The listing builds one solid part. Answer for the finished solid, in the listing's coordinates (mm). A direction names the side the tool comes from. Give positions to 0.01 mm unless a question says otherwise; leave off trailing zeros. Write each loop counter-clockwise with the first axis right and the second up, starting at its lowest first coordinate (ties: lowest second). Pieces come first, ordered by that corner, then holes. Notation, with made-up numbers: (66, -16) -> (85, -16) arc R19 cw to (85, -9) -> close; hole circle Ø1 at (71.25, -21.75). An arc over 180 degrees is marked (long way). Put each result on its own line as item: value. Start each with the question number.
1) For faces 4 (the flat face through (8.699, 13, 8)), 5 (the flat face through (-13, 9.5, -12)), 6 (the flat face through (-13, 5, 6.329)), determine the directions among +Z, -Z, +X, -X, +Y, -Y from which every point of the face is accessible in a straight line to the end or side of a thin tool.
2) A cutting plane is placed at A-A (z = -10.5). Write down the section's boundary in (x, y), then the cut area to 3 significant figures.
3) A cutting plane is placed at C-C (z = 5.5). Write down the section's boundary in (x, y), then the cut area to 3 significant figures.
4) Find the intervals of material crossed by line 1 along Z through (x, y) = (-1.5, 9); line 2 along Z through (x, y) = (-6, 18.5); line 3 along X through (y, z) = (4.5, -12.5), in increasing order. Write a range as from..to.
5) A cutting plane is placed at B-B (x = -23.5). Write down the section's boundary in (y, z), then the cut area to 3 significant figures.
6) For a pull along Y with two mould halves and no side action, classify faces 1 (the flat face through (12, 2, -7)), 2 (the cylindrical face through (6.674, 30.573, -1.74)), 3 (the flat face through (4.699, 4, -14)) as released by +Y, released by -Y, zero draft, split by the parting line, or undercut.
7) Flat-ended cylindrical pins translate along their axes: pin 1 Ø10 at (x, z) = (18, 10.5) entering from +Y; pin 2 Ø1.5 at (x, z) = (-13, 2.5) entering from -Y; pin 3 Ø8 at (x, y) = (11.5, 25.5) entering from +Z. Find the tip coordinate at first contact, or state that the pin passes through.
from build123d import *

# Parameters (mm, degrees)
SKETCH1_W           = 48
SKETCH1_H           = 27.75
BOSS_EXTRUDE1_DEPTH = 31
CUT_EXTRUDE1_DEPTH  = 36
SKETCH3_W           = 22
SKETCH3_H           = 25.75
CUT_EXTRUDE2_DEPTH  = 29
CUT_EXTRUDE3_DEPTH  = 45.957983893
BOSS_EXTRUDE2_START = -26
SKETCH5_W           = 27.75
SKETCH5_H           = 17
BOSS_EXTRUDE2_DEPTH = 41
SKETCH10_W          = 27.75
SKETCH10_H          = 23
BOSS_EXTRUDE4_DEPTH = 8
CHAMFER1_SIZE       = 38
CHAMFER1_SIZE2      = 10
FILLET1_R           = 10
SKETCH6_W           = 9
SKETCH6_H           = 9.5
CUT_EXTRUDE4_DEPTH  = 8
BOSS_EXTRUDE3_DEPTH = 18
SKETCH8_R           = 1.375
CUT_EXTRUDE5_DEPTH  = 17
SKETCH9_W           = 6
SKETCH9_H           = 10
CUT_EXTRUDE6_DEPTH  = 9


with BuildPart() as part:
    # Sketch1 → Boss-Extrude1 (new body)
    with BuildSketch(Plane(origin=(0, 0, 0), x_dir=(1, 0, 0), z_dir=(0, 1, 0))):
        with Locations((6.698630137, 1.546232877)):
            Rectangle(SKETCH1_W, SKETCH1_H)
    extrude(amount=BOSS_EXTRUDE1_DEPTH)

    # Sketch2 → Cut-Extrude1 (cut)
    with BuildSketch(Plane.ZY.offset(17.301369863)):
        Polygon((-7.921232877, 25.25), (4.828767123, 25.25), (4.828767123, 2), (2.703767123, 2), (2.703767123, 0), (-5.796232877, 0), (-5.796232877, 2), (-7.921232877, 2), align=None)
    extrude(amount=-CUT_EXTRUDE1_DEPTH, mode=Mode.SUBTRACT)

    # Sketch3 → Cut-Extrude2 (cut)
    with BuildSketch(Plane(origin=(0, 31, 0), x_dir=(1, 0, 0), z_dir=(0, 1, 0))):
        with Locations((19.698630137, 1.546232877)):
            Rectangle(SKETCH3_W, SKETCH3_H)
    extrude(amount=-CUT_EXTRUDE2_DEPTH, mode=Mode.SUBTRACT)

    # Sketch4 → Cut-Extrude3 (cut, through all)
    with BuildSketch(Plane(origin=(0, 2, 0), x_dir=(1, 0, 0), z_dir=(0, 1, 0))):
        with BuildLine():
            Line((20.698630137, -1.953767123), (18.698630137, -1.953767123))
            ThreePointArc((18.698630137, -1.953767123), (15.198630137, 1.546232877), (18.698630137, 5.046232877))
            Line((18.698630137, 5.046232877), (20.698630137, 5.046232877))
            ThreePointArc((20.698630137, 5.046232877), (24.198630137, 1.546232877), (20.698630137, -1.953767123))
        make_face()
    extrude(amount=-CUT_EXTRUDE3_DEPTH, mode=Mode.SUBTRACT)

    # Sketch5 → Boss-Extrude2 (add)
    with BuildSketch(Plane.ZY.offset(17.301369863).offset(BOSS_EXTRUDE2_START)):
        with Locations((-1.546232877, 33.75)):
            Rectangle(SKETCH5_W, SKETCH5_H)
    extrude(amount=BOSS_EXTRUDE2_DEPTH)

    # Sketch10 → Boss-Extrude4 (add)
    with BuildSketch(Plane.ZY.offset(32.301369863)):
        with Locations((-1.546232877, 30.75)):
            Rectangle(SKETCH10_W, SKETCH10_H)
    extrude(amount=-BOSS_EXTRUDE4_DEPTH)

    # Chamfer1
    chamfer1_edges = [part.edges().sort_by_distance(p)[0] for p in [
        (8.698630137, 42.25, -1.546232877),
    ]]
    chamfer1_side = [part.faces().sort_by_distance(p)[0] for p in [
        (-11.801369863, 42.25, -1.546232877),
    ]]
    chamfer(chamfer1_edges, length=CHAMFER1_SIZE, length2=CHAMFER1_SIZE2, reference=chamfer1_side[0])

    # Fillet1
    # the kernel refuses this fillet: 10 mm, written as the material it takes off along each edge
    with BuildSketch(Plane(origin=(30.698630137, 31, -40.421232877), x_dir=(-1, 0, 0), z_dir=(0, 0, 1))) as fillet1_piece_1:
        with BuildLine():
            CenterArc((FILLET1_R, FILLET1_R), FILLET1_R, 180, 90)
            Line((0, FILLET1_R), (0, 0))
            Line((0, 0), (FILLET1_R, 0))
        make_face()
    extrude(amount=51, mode=Mode.SUBTRACT)
    with BuildSketch(Plane(origin=(30.698630137, 31, -13.671232877), x_dir=(0, -1, 0), z_dir=(0, 0, 1))) as fillet1_piece_2:
        with BuildLine():
            CenterArc((FILLET1_R, -FILLET1_R), FILLET1_R, 90, 90)
            Line((0, -FILLET1_R), (0, 0))
            Line((0, 0), (FILLET1_R, 0))
        make_face()
    extrude(amount=51, mode=Mode.SUBTRACT)
    with BuildSketch(Plane(origin=(8.698630137, 32.25, -34.693446961), x_dir=(-0.9670745372626461, 0.25449329927964454, 0), z_dir=(0, 0, 1))) as fillet1_piece_3_section:
        with BuildLine():
            CenterArc((FILLET1_R * 0.770888563389, FILLET1_R), FILLET1_R, 194.743562836, 75.256437164)
            Line((-FILLET1_R * 0.196185973874, FILLET1_R * 0.74550670072), (0, 0))
            Line((0, 0), (FILLET1_R * 0.770888563389, 0))
        make_face()
    fillet1_piece_3 = extrude(amount=66.294428169, mode=Mode.PRIVATE)
    fillet1_piece_3 = split(fillet1_piece_3, bisect_by=Plane(origin=(6.418470389, 31, -14.921232877), z_dir=(0, 1, 0)), keep=Keep.TOP, mode=Mode.PRIVATE)
    add(fillet1_piece_3, mode=Mode.SUBTRACT)
    with BuildSketch(Plane(origin=(8.698630137, 32.25, -34.693446961), x_dir=(-0.9670745372626461, 0.25449329927964454, 0), z_dir=(0, 0, 1))) as fillet1_piece_4_section:
        with BuildLine():
            CenterArc((FILLET1_R * 0.770888563389, FILLET1_R), FILLET1_R, 194.743562836, 75.256437164)
            Line((-FILLET1_R * 0.196185973874, FILLET1_R * 0.74550670072), (0, 0))
            Line((0, 0), (FILLET1_R * 0.770888563389, 0))
        make_face()
    fillet1_piece_4 = extrude(amount=66.294428169, mode=Mode.PRIVATE)
    fillet1_piece_4 = split(fillet1_piece_4, bisect_by=Plane(origin=(8.005221355, 29.431341636, -14.421232877), z_dir=(0, 0, 1)), keep=Keep.TOP, mode=Mode.PRIVATE)
    fillet1_piece_4 = split(fillet1_piece_4, bisect_by=Plane(origin=(8.005221355, 29.431341636, 11.328767123), z_dir=(0, 0, -1)), keep=Keep.TOP, mode=Mode.PRIVATE)
    add(fillet1_piece_4, mode=Mode.SUBTRACT)

    # Sketch6 → Cut-Extrude4 (cut)
    with BuildSketch(Plane.ZY.offset(17.301369863)):
        with Locations((10.828767123, 4.75)):
            Rectangle(SKETCH6_W, SKETCH6_H)
    cut_extrude4 = extrude(amount=-CUT_EXTRUDE4_DEPTH, mode=Mode.SUBTRACT)

    # Sketch7 → Boss-Extrude3 (add)
    with BuildSketch(Plane.ZY.offset(9.301369863)):
        Polygon((12.328767123, 0), (12.328767123, 9.5), (12.328767123, 14.5), (15.328767123, 14.5), (15.328767123, 9.5), (15.328767123, 0), (15.328767123, -0.5), (6.328767123, -0.5), (6.328767123, 0), align=None)
    boss_extrude3 = extrude(amount=-BOSS_EXTRUDE3_DEPTH)

    # Sketch8 → Cut-Extrude5 (cut)
    with BuildSketch(Plane.ZY.offset(9.301369863)):
        with Locations((12.328767123, 2)):
            Circle(SKETCH8_R)
    cut_extrude5 = extrude(amount=-CUT_EXTRUDE5_DEPTH, mode=Mode.SUBTRACT)

    # Sketch9 → Cut-Extrude6 (cut)
    with BuildSketch(Plane.XY.offset(15.328767123)):
        with Locations((1.698630137, 4.5)):
            Rectangle(SKETCH9_W, SKETCH9_H)
    cut_extrude6 = extrude(amount=-CUT_EXTRUDE6_DEPTH, mode=Mode.SUBTRACT)

    # Mirror1: Cut-Extrude4, Boss-Extrude3, Cut-Extrude5, Cut-Extrude6 across plane
    add(cut_extrude4.mirror(Plane.XY.offset(-1.546232877)), mode=Mode.SUBTRACT)
    add(boss_extrude3.mirror(Plane.XY.offset(-1.546232877)))
    add(cut_extrude5.mirror(Plane.XY.offset(-1.546232877)), mode=Mode.SUBTRACT)
    add(cut_extrude6.mirror(Plane.XY.offset(-1.546232877)), mode=Mode.SUBTRACT)


solid = part.part
Reply:
1. face 4: +X, +Y
1. face 5: -Z, -X, -Y
1. face 6: +Z, -X, -Y
2. outline: (-32.3, 19.25) -> (-24.3, 19.25) -> (-24.3, 25.25) -> (-17.3, 25.25) -> (-17.3, 9.5) -> (-9.3, 9.5) -> (-9.3, -0.5) -> (-1.3, -0.5) -> (-1.3, 9.5) -> (4.7, 9.5) -> (4.7, -0.5) -> (8.7, -0.5) -> (8.7, 0) -> (30.7, 0) -> (30.7, 2) -> (8.7, 2) -> (8.7, 24.54) arc R10 ccw to (1.24, 34.21) -> (-29.3, 42.25) -> (-32.3, 42.25) -> close
2. area: 1,120 mm2
3. outline: (-32.3, 19.25) -> (-24.3, 19.25) -> (-24.3, 25.25) -> (-17.3, 25.25) -> (-17.3, 0) -> (30.7, 0) -> (30.7, 2) -> (8.7, 2) -> (8.7, 24.54) arc R10 ccw to (1.24, 34.21) -> (-29.3, 42.25) -> (-32.3, 42.25) -> close
3. area: 1,240 mm2
4. line 1: z = -18.42..-7.92, 4.83..15.33
4. line 2: z = -15.42..-7.92, 4.83..12.33
4. line 3: x = -9.3..-1.3, 4.7..8.7
5. outline: (25.25, -15.42) -> (40.72, -15.42) -> (40.72, 12.33) -> (25.25, 12.33) -> close
5. area: 429 mm2
6. face 1: undercut
6. face 2: released by +Y
6. face 3: zero draft
7. pin 1: stops at y = 31
7. pin 2: stops at y = 0
7. pin 3: stops at z = 12.33
